Work out the finished part from the listing and answer in its coordinate system (mm). Face numbers are marked on the shaded views. A direction names the side the tool comes from. Round coordinates to 2 decimals unless told otherwise and drop trailing zeros. Loops run counter-clockwise (first coordinate to the right, second up) from the corner with the lowest first, then second, coordinate; pieces in that order, holes last. Notation, with made-up numbers: (-0.75, 68) - (40.25, 68) arc R30 ccw to (40.25, 101) - close; hole circle Ø10 at (-24.75, 75.25). An arc over 180 degrees is marked (long way). Use CSV: the item, a comma, the result in double quotes. Start each with the question number.
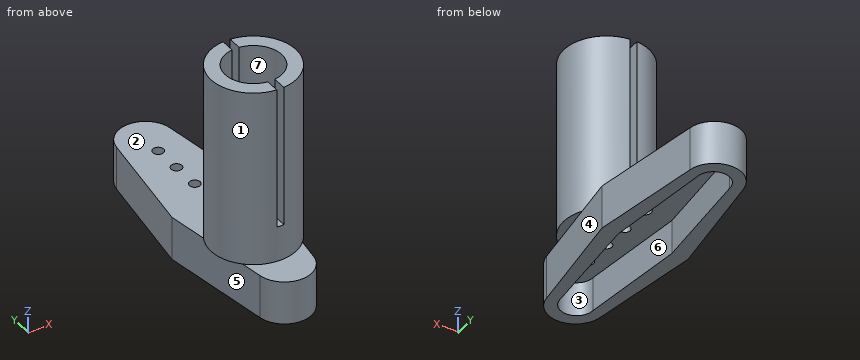
from build123d import *

# Parameters (mm, degrees)
BOSS_EXTRUDE1_DEPTH     = 6
CUT_EXTRUDE3_DEPTH      = 4.7
CUT_EXTRUDE4_DEPTH      = 21.471687766
CUT_EXTRUDE4_DEPTH_BACK = 21.471687766
SKETCH4_R               = 0.75
SKETCH6_R               = 0.75
CUT_EXTRUDE6_DEPTH      = 21.471687766
LPATTERN1_COUNT         = 3
LPATTERN1_PITCH         = 4
SCALE1_SCALE            = 1.02
SKETCH7_W               = 12.24
SKETCH7_H               = 6.12
CUT_EXTRUDE7_DEPTH      = 22.106506047
SKETCH8_R               = 0.875
CUT_EXTRUDE8_DEPTH      = 22.121773144
SKETCH9_R               = 6
SKETCH9_R_2             = 4
BOSS_EXTRUDE2_DEPTH     = 25
SKETCH10_W              = 1
SKETCH10_H              = 40
CUT_EXTRUDE9_DEPTH      = 38.052107321


with BuildPart() as part:
    # Sketch2 → Boss-Extrude1 (new body)
    with BuildSketch(Plane.XY):
        with BuildLine():
            Line((-6, 0), (-3.720572803, -15.718868867))
            ThreePointArc((-3.720572803, -15.718868867), (-5.969e-06, -19), (3.720571311, -15.71888071))
            Line((3.720571311, -15.71888071), (6, 0))
            ThreePointArc((6, 0), (0, 6), (-6, 0))
        make_face()
    extrude(amount=BOSS_EXTRUDE1_DEPTH)

    # Sketch3 → Cut-Extrude3 (cut)
    with BuildSketch(Plane.XY):
        with BuildLine():
            Line((-3.75, 0), (-2.25, -15))
            ThreePointArc((-2.25, -15), (0, -17.25), (2.25, -15))
            Line((2.25, -15), (3.75, 0))
            ThreePointArc((3.75, 0), (0, 3.75), (-3.75, 0))
        make_face()
    extrude(amount=CUT_EXTRUDE3_DEPTH, mode=Mode.SUBTRACT)

    # Sketch4 → Cut-Extrude4 (cut, two sides: drawn at the far end of the back side and taken through both)
    with BuildSketch(Plane(origin=(0, 0, 4.7), x_dir=(-1, 0, 0), z_dir=(0, 0, -1)).offset(-CUT_EXTRUDE4_DEPTH_BACK)):
        Circle(SKETCH4_R)
    extrude(amount=CUT_EXTRUDE4_DEPTH + CUT_EXTRUDE4_DEPTH_BACK, mode=Mode.SUBTRACT)

    # Sketch6 → Cut-Extrude6 (cut, symmetric)
    with BuildSketch(Plane(origin=(0, 0, 4.7), x_dir=(-1, 0, 0), z_dir=(0, 0, -1))):
        with Locations((0, -4.5)):
            Circle(SKETCH6_R)
    cut_extrude6 = extrude(amount=CUT_EXTRUDE6_DEPTH, both=True, mode=Mode.SUBTRACT)

    # LPattern1: Cut-Extrude6 ×3
    with Locations(*[(0, -i * LPATTERN1_PITCH, 0) for i in range(1, LPATTERN1_COUNT)]):
        add(cut_extrude6, mode=Mode.SUBTRACT)


with BuildPart() as part_1:
    # Scale1: scaled about (6e-08, -5.397561761, 3.434577722)
    add(part.part.scale(SCALE1_SCALE).moved(Location((-1e-09, 0.107951235, -0.068691554))))

    # Sketch7 → Cut-Extrude7 (cut, through all)
    with BuildSketch(Plane(origin=(0, 0, 0), x_dir=(1, 0, 0), z_dir=(0, 1, 0))):
        with Locations((-1e-09, -2.991308446)):
            Rectangle(SKETCH7_W, SKETCH7_H)
    extrude(amount=CUT_EXTRUDE7_DEPTH, mode=Mode.SUBTRACT)

    # Mirror3: part across plane


with BuildPart() as part_2:
    add(part_1.part)
    add(part_1.part.mirror(Plane.ZX))

    # Sketch8 → Cut-Extrude8 (cut, through all)
    with BuildSketch(Plane.XY.offset(6.051308446)):
        Circle(SKETCH8_R)
    extrude(amount=-CUT_EXTRUDE8_DEPTH, mode=Mode.SUBTRACT)

    # Sketch9 → Boss-Extrude2 (add)
    with BuildSketch(Plane.XY.offset(6.051308446)):
        with Locations(Location((-1e-09, -8.562048765, 0), (0, 0, 151.579121381))):
            Circle(SKETCH9_R)
        with Locations(Location((-1e-09, -8.562048765, 0), (0, 0, 100.806376462))):
            Circle(SKETCH9_R_2, mode=Mode.SUBTRACT)
    extrude(amount=BOSS_EXTRUDE2_DEPTH)

    # Sketch10 → Cut-Extrude9 (cut, through all)
    with BuildSketch(Plane(origin=(0, 0, 0), x_dir=(1, 0, 0), z_dir=(0, 1, 0))):
        with Locations((0, -31.051308446)):
            Rectangle(SKETCH10_W, SKETCH10_H)
    extrude(amount=-CUT_EXTRUDE9_DEPTH, mode=Mode.SUBTRACT)


solid = part_2.part
Item 1: A cutting plane is placed at D-D (x = 4.75). Determine the outline of the cut face in (y, z).
Item 2: A cutting plane is placed at C-C (x = 0). State how many separate pieces and enclosed holes the cut face has, plus the area to 3 significant figures.
Item 3: Find the intervals of material crossed by probe 1 along Z at (x, y) = (0.25, -4); probe 2 along Z at (x, y) = (-2, 7); probe 3 along X at (y, z) = (-11, 19.5), in increasing order. Write a range as [from, to].
Item 4: Each of these flat-tipped pins is pushed along its axis until it touches: pin 1 Ø6 at (x, y) = (-3.5, 10.5) entering from +Z; pin 2 Ø1 at (x, y) = (1.5, 11.5) entering from -Z; pin 3 Ø4 at (y, z) = (-3, 3.5) entering from -X. Where does it stop, or does it pass through?
Item 5: Which of the six approach directions +Z, -Z, +X, -X, +Y, -Y give full straight-line access (tool end or side, diameter ignored) to the marked faces 5, 6 and 7?
Item 6: A cutting plane is placed at B-B (z = 2). Determine the outline of the cut face in (x, y) (3 decimals).
Item 7: The mould has two halves that part along Y. Classify the marked faces 1, 2, 3 and 4: pulls with the +Y half, pulls with the -Y half, needs draft (parallel to the pull), parting line crosses it, or undercut.
Item 8: A cutting plane is placed at A-A (z = 24.5). Determine the outline of the cut face in (x, y), plus the area to 3 significant figures.
Result sheet:
1,outline,"(-12.23, 6.05) - (-9.34, 6.05) - (-9.34, -0.07) - (9.34, -0.07) - (9.34, 6.05) - (-4.9, 6.05) - (-4.9, 31.05) - (-12.23, 31.05) - close"
2,separate pieces,"8"
2,enclosed holes,"0"
2,area,"73.7 mm^2"
3,probe 1,"[6.05, 11.05]"
3,probe 2,"[4.73, 6.05]"
3,probe 3,"[-5.48, -3.17], [3.17, 5.48]"
4,pin 1,"z = 6.05"
4,pin 2,"z = 4.73"
4,pin 3,"x = -5.96"
5,face 5,"-Z, -X, -Y"
5,face 6,"-Z"
5,face 7,"+Z"
6,outline,"(-6.104, 0) - (-3.795, -15.925) arc R3.825 ccw to (3.795, -15.925) - (6.104, 0) - (3.795, 15.925) arc R3.825 ccw to (-3.795, 15.925) - close; hole (-3.814, 0) - (-2.295, -15.192) arc R2.295 ccw to (2.295, -15.192) - (3.814, 0) - (2.295, 15.192) arc R2.295 ccw to (-2.295, 15.192) - close"
7,face 1,"parting line crosses it"
7,face 2,"needs draft"
7,face 3,"undercut"
7,face 4,"pulls with the -Y half"
8,outline,"(-0.5, -14.54) - (-0.5, -12.53) arc R4 cw to (-0.5, -4.59) - (-0.5, -2.58) arc R6 ccw to start; (0.5, -14.54) arc R6 ccw to (0.5, -2.58) - (0.5, -4.59) arc R4 cw to (0.5, -12.53) - close"
8,area,"58.8 mm^2"
